from build123d import *

# Parameters (mm, degrees)
BOSS_EXTRUDE1_DEPTH = 5
BOSS_EXTRUDE3_DEPTH = 5
SKETCH5_W           = 5
SKETCH5_H           = 42
BOSS_EXTRUDE4_DEPTH = 33
SKETCH6_W           = 5
SKETCH6_H           = 42
BOSS_EXTRUDE5_DEPTH = 5
SKETCH7_W           = 5
SKETCH7_H           = 42
BOSS_EXTRUDE6_DEPTH = 130


with BuildPart() as part:
    # Sketch2 → Boss-Extrude1 (new body)
    with BuildSketch(Plane(origin=(0, 0, 0), x_dir=(0, 0, -1), z_dir=(1, 0, 0))):
        Polygon((-21, 16.4), (-21, -16.4), (-16.4, -21), (16.4, -21), (21, -16.4), (21, 16.4), (16.4, 21), (-16.4, 21), align=None)
        with BuildLine():
            ThreePointArc((-14, 15.5), (-15.5, 17), (-17, 15.5))
            ThreePointArc((-17, 15.5), (-15.5, 14), (-14, 15.5))
        make_face(mode=Mode.SUBTRACT)
        with BuildLine():
            ThreePointArc((15.75, 0), (0, 15.75), (-15.75, 0))
            ThreePointArc((-15.75, 0), (0, -15.75), (15.75, 0))
        make_face(mode=Mode.SUBTRACT)
        with BuildLine():
            ThreePointArc((17, -15.5), (15.5, -14), (14, -15.5))
            ThreePointArc((14, -15.5), (15.5, -17), (17, -15.5))
        make_face(mode=Mode.SUBTRACT)
        with BuildLine():
            ThreePointArc((17, 15.5), (15.5, 17), (14, 15.5))
            ThreePointArc((14, 15.5), (15.5, 14), (17, 15.5))
        make_face(mode=Mode.SUBTRACT)
        with BuildLine():
            ThreePointArc((-14, -15.5), (-15.5, -14), (-17, -15.5))
            ThreePointArc((-17, -15.5), (-15.5, -17), (-14, -15.5))
        make_face(mode=Mode.SUBTRACT)
    extrude(amount=BOSS_EXTRUDE1_DEPTH)

    # Sketch4 → Boss-Extrude3 (add)
    with BuildSketch(Plane(origin=(5, 0, 0), x_dir=(0, 0, -1), z_dir=(1, 0, 0))):
        Polygon((26, 21), (26, -21), (16.4, -21), (21, -16.4), (21, 16.4), (16.4, 21), align=None)
    extrude(amount=-BOSS_EXTRUDE3_DEPTH)

    # Sketch5 → Boss-Extrude4 (add)
    with BuildSketch(Plane.ZY):
        with Locations((-23.5, 0)):
            Rectangle(SKETCH5_W, SKETCH5_H)
    extrude(amount=BOSS_EXTRUDE4_DEPTH)

    # Sketch6 → Boss-Extrude5 (add)
    with BuildSketch(Plane.ZY.offset(33)):
        with Locations((-23.5, 0)):
            Rectangle(SKETCH6_W, SKETCH6_H)
        Polygon((21, 16.4), (16.4, 21), (-21, 21), (-21, -21), (16.4, -21), (21, -16.4), align=None)
    extrude(amount=BOSS_EXTRUDE5_DEPTH)

    # Sketch7 → Boss-Extrude6 (add)
    with BuildSketch(Plane(origin=(5, 0, 0), x_dir=(0, 0, -1), z_dir=(1, 0, 0))):
        with Locations((23.5, 0)):
            Rectangle(SKETCH7_W, SKETCH7_H)
    extrude(amount=BOSS_EXTRUDE6_DEPTH)


solid = part.part
Geometry check sheet. Reference: the model listing, model coordinates, mm. A direction names the side the tool comes from. Give positions to 0.01 mm unless a question says otherwise; leave off trailing zeros. Loops run counter-clockwise (first coordinate to the right, second up) from the corner with the lowest first, then second, coordinate; pieces in that order, holes last.
(1) Release check for a two-part mould opening along Y. For faces 5 (the flat face through (0, 14, 9)), 6 (the flat face through (-35.5, 18.7, 18.7)), 7 (the cylindrical face through (2.46, 15.43, -17)) record: released by +Y, released by -Y, zero draft, split by the parting line, or undercut.
From the geometry:
face 5: zero draft
face 6: released by +Y
face 7: undercut
(2) Section check A-A on z = -18.5. Record the cut outline in (x, y), then the cut area to 3 significant figures.
From the geometry:
outline: (-38, -21) - (-33, -21) - (-33, 21) - (-38, 21) - close; (0, -21) - (5, -21) - (5, 21) - (0, 21) - close
area: 420 mm2
(3) Section check B-B on z = 0. Record the cut outline in (x, y).
From the geometry:
outline: (-38, -21) - (-33, -21) - (-33, 21) - (-38, 21) - close; (0, -21) - (5, -21) - (5, -15.75) - (0, -15.75) - close; (0, 15.75) - (5, 15.75) - (5, 21) - (0, 21) - close
(4) Set-up check for faces 1 (the flat face through (69, 0, -21)), 2 (the cylindrical face through (2.465, -15.616, -2.05)), 3 (the flat face through (29, 21, -22)), 4 (the flat face through (-16, 0, -21)): record each of +Z, -Z, +X, -X, +Y, -Y from which the full face is reachable in a straight line by a thin tool's end or side.
From the geometry:
face 1: +Z, +X, +Y, -Y
face 2: +X
face 3: +Z, -Z, +X, -X, +Y
face 4: +Z, +Y, -Y
(5) Depth check by flat-ended pin: pin 1 Ø4 at (x, y) = (94.5, -5) entering from +Z; pin 2 Ø3 at (y, z) = (12.5, 13) entering from +X; pin 3 Ø6 at (y, z) = (-11.5, -5) entering from +X. Enter the tip coordinate at first touch or a pass-through.
From the geometry:
pin 1: stops at z = -21
pin 2: stops at x = 5
pin 3: stops at x = -33
(6) Thickness scan on L1, parallel to X at y = 19, z = 10.5; L2, parallel to Y at x = 2, z = 0; L3, parallel to X at y = -2.5, z = -7.5. Record the ranges inside material, lowest first.
From the geometry:
L1: x = -38 to -33, 0 to 5
L2: y = -21 to -15.75, 15.75 to 21
L3: x = -38 to -33
(7) Section check D-D on x = 87. Record the cut outline in (y, z).
From the geometry:
outline: (-21, -26) - (21, -26) - (21, -21) - (-21, -21) - close
(8) Section check C-C on y = 3. Record the cut outline in (x, z), then the cut area to 3 significant figures.
From the geometry:
outline: (-38, -26) - (135, -26) - (135, -21) - (5, -21) - (5, -15.46) - (0, -15.46) - (0, -21) - (-33, -21) - (-33, 21) - (-38, 21) - close; (0, 15.46) - (5, 15.46) - (5, 21) - (0, 21) - close
area: 1,130 mm2
